from build123d import *

# Parameters (mm, degrees)
SCHIZZO1_W                   = 27
SCHIZZO1_H                   = 32
ESTRUSIONE_ESTRUSIONE1_DEPTH = 31
SCHIZZO2_R                   = 1.75
TAGLIO_ESTRUSIONE1_DEPTH     = 32
SCHIZZO8_OUTSIDE_W           = 39.42
SCHIZZO8_OUTSIDE_H           = 43.42
SCHIZZO8_OUTSIDE_W_2         = 27
SCHIZZO8_OUTSIDE_H_2         = 25
TAGLIO_ESTRUSIONE7_DEPTH     = 33
SCHIZZO10_R                  = 5
TAGLIO_ESTRUSIONE8_DEPTH     = 1.5
SCHIZZO11_R                  = 4
TAGLIO_ESTRUSIONE9_DEPTH     = 33
SCHIZZO12_R                  = 5
TAGLIO_ESTRUSIONE10_DEPTH    = 1.5


with BuildPart() as part:
    # Schizzo1 → Estrusione-Estrusione1 (new body)
    with BuildSketch(Plane.XY):
        Rectangle(SCHIZZO1_W, SCHIZZO1_H)
    extrude(amount=ESTRUSIONE_ESTRUSIONE1_DEPTH)

    # Schizzo2 → Taglio-Estrusione1 (cut, through all)
    with BuildSketch(Plane(origin=(0, 0, 0), x_dir=(-1, 0, 0), z_dir=(0, 0, -1))):
        with Locations((-10, 7.5)):
            Circle(SCHIZZO2_R)
        with Locations((10, 7.5)):
            Circle(SCHIZZO2_R)
        with Locations((10, -7.5)):
            Circle(SCHIZZO2_R)
        with Locations((-10, -7.5)):
            Circle(SCHIZZO2_R)
    extrude(amount=-TAGLIO_ESTRUSIONE1_DEPTH, mode=Mode.SUBTRACT)

    # Schizzo8 outside → Taglio-Estrusione7 (cut, through all)
    with BuildSketch(Plane(origin=(0, 16, 0), x_dir=(1, 0, 0), z_dir=(0, 1, 0))):
        with Locations((0, -15.5)):
            Rectangle(SCHIZZO8_OUTSIDE_W, SCHIZZO8_OUTSIDE_H)
        with Locations((0, -18.5)):
            Rectangle(SCHIZZO8_OUTSIDE_W_2, SCHIZZO8_OUTSIDE_H_2, mode=Mode.SUBTRACT)
    extrude(amount=-TAGLIO_ESTRUSIONE7_DEPTH, mode=Mode.SUBTRACT)

    # Schizzo10 → Taglio-Estrusione8 (cut)
    with BuildSketch(Plane(origin=(0, 16, 0), x_dir=(1, 0, 0), z_dir=(0, 1, 0))):
        with Locations((0, -16.5)):
            Circle(SCHIZZO10_R)
    extrude(amount=-TAGLIO_ESTRUSIONE8_DEPTH, mode=Mode.SUBTRACT)

    # Schizzo11 → Taglio-Estrusione9 (cut, through all)
    with BuildSketch(Plane(origin=(0, 16, 0), x_dir=(1, 0, 0), z_dir=(0, 1, 0))):
        with Locations((0, -16.5)):
            Circle(SCHIZZO11_R)
    extrude(amount=-TAGLIO_ESTRUSIONE9_DEPTH, mode=Mode.SUBTRACT)

    # Schizzo12 → Taglio-Estrusione10 (cut)
    with BuildSketch(Plane.XZ.offset(16)):
        with Locations((0, 16.5)):
            Circle(SCHIZZO12_R)
    extrude(amount=-TAGLIO_ESTRUSIONE10_DEPTH, mode=Mode.SUBTRACT)


solid = part.part
Source: CAD feature listing. Evaluate the final solid. Frame: model axes, mm. A direction names the side the tool comes from. Round coordinates to 2 decimals unless told otherwise and drop trailing zeros. Loops run counter-clockwise (first coordinate to the right, second up) from the corner with the lowest first, then second, coordinate; pieces in that order, holes last. Notation, with made-up numbers: M 29,6 L 59,6 A21 cw 59,38 Z; hole C -15.5,20 d4. An arc over 180 degrees is marked long. Return JSON: item names as keys, results as strings. Group by question number.
1. Section query A-A on y = 7.5. Output: boundary loops of the cut face in (x, z), and give its area (3 significant figures).
2. Section query B-B on z = 16.5. Output: boundary loops of the cut face in (x, y), and give its area (3 significant figures).
3. Reachability of faces 4 (the face through (-10.81, -9.05, 18.32)), 5 (the face through (-4, 14.5, 18)), 6 (the face through (-4, -14.5, 15)) from +Z, -Z, +X, -X, +Y, -Y: full face, straight path, thin tool, end or side. Return the list, or none.
4. Section query C-C on x = 10. Output: boundary loops of the cut face in (y, z).
5. Material intervals for line 1 along Y through (x, z) = (-10, 20); line 2 along Z through (x, y) = (0, 15.35); line 3 along X through (y, z) = (8, 15.25), sorted ascending. Write a range as from..to.
6. Section query D-D on x = 0. Output: boundary loops of the cut face in (y, z), and give its area (3 significant figures).
7. Pin query (flat end, axial travel): pin 1 (9 mm diameter, centred on x = 0, z = 16.5, fed in from +Y); pin 2 (9 mm diameter, centred on x = 0, z = 16.5, fed in from -Y). Return the tip coordinate at first contact, or that it passes through.
8. Mould query, pull axis Z, two halves, no side actions, for faces 1 (the face through (3, -16, 21)), 2 (the face through (-1.08, -15.26, 11.62)), 3 (the face through (0, 0, 6)). Classes: released by +Z, released by -Z, zero draft, split by the parting line, or undercut.
Checks:
{
 "1": {"outline": "M -13.5,6 L -11.75,6 L -11.75,31 L -13.5,31 Z; M -8.25,6 L 8.25,6 L 8.25,31 L -8.25,31 Z; M 11.75,6 L 13.5,6 L 13.5,31 L 11.75,31 Z; hole C 0,16.5 d8", "area": "450 mm²"},
 "2": {"outline": "M -13.5,-16 L -5,-16 L -5,-14.5 L -4,-14.5 L -4,14.5 L -5,14.5 L -5,16 L -13.5,16 Z; M 4,-14.5 L 5,-14.5 L 5,-16 L 13.5,-16 L 13.5,16 L 5,16 L 5,14.5 L 4,14.5 Z; hole C -10,-7.5 d3.5; hole C -10,7.5 d3.5; hole C 10,-7.5 d3.5; hole C 10,7.5 d3.5", "area": "564 mm²"},
 "3": {"face 4": "+Z, -Z", "face 5": "+Y", "face 6": "-Y"},
 "4": {"outline": "M -16,6 L -9.25,6 L -9.25,31 L -16,31 Z; M -5.75,6 L 5.75,6 L 5.75,31 L -5.75,31 Z; M 9.25,6 L 16,6 L 16,31 L 9.25,31 Z"},
 "5": {"line 1": "y = -16..-9.25, -5.75..5.75, 9.25..16", "line 2": "z = 6..11.5, 21.5..31", "line 3": "x = -13.5..-11.68, -8.32..-3.8, 3.8..8.32, 11.68..13.5"},
 "6": {"outline": "M -16,6 L 16,6 L 16,11.5 L 14.5,11.5 L 14.5,12.5 L -14.5,12.5 L -14.5,11.5 L -16,11.5 Z; M -16,21.5 L -14.5,21.5 L -14.5,20.5 L 14.5,20.5 L 14.5,21.5 L 16,21.5 L 16,31 L -16,31 Z", "area": "538 mm²"},
 "7": {"pin 1": "stops at y = 14.5", "pin 2": "stops at y = -14.5"},
 "8": {"face 1": "zero draft", "face 2": "undercut", "face 3": "released by -Z"}
}
